Geometry: see drawing. Coordinates: mm, zero at the bounding-box minimum. Give positions to 0.01 mm unless a question says otherwise; leave off trailing zeros. Loops run counter-clockwise (first coordinate to the right, second up) from the corner with the lowest first, then second, coordinate; pieces in that order, holes last. Notation, with made-up numbers: (12.25, 66.25) -> (70.25, 66.25) arc R26 ccw to (70.25, 87.25) -> close; hole circle Ø5 at (67, 72). An arc over 180 degrees is marked (long way). One line per question, with ' | ' between items.
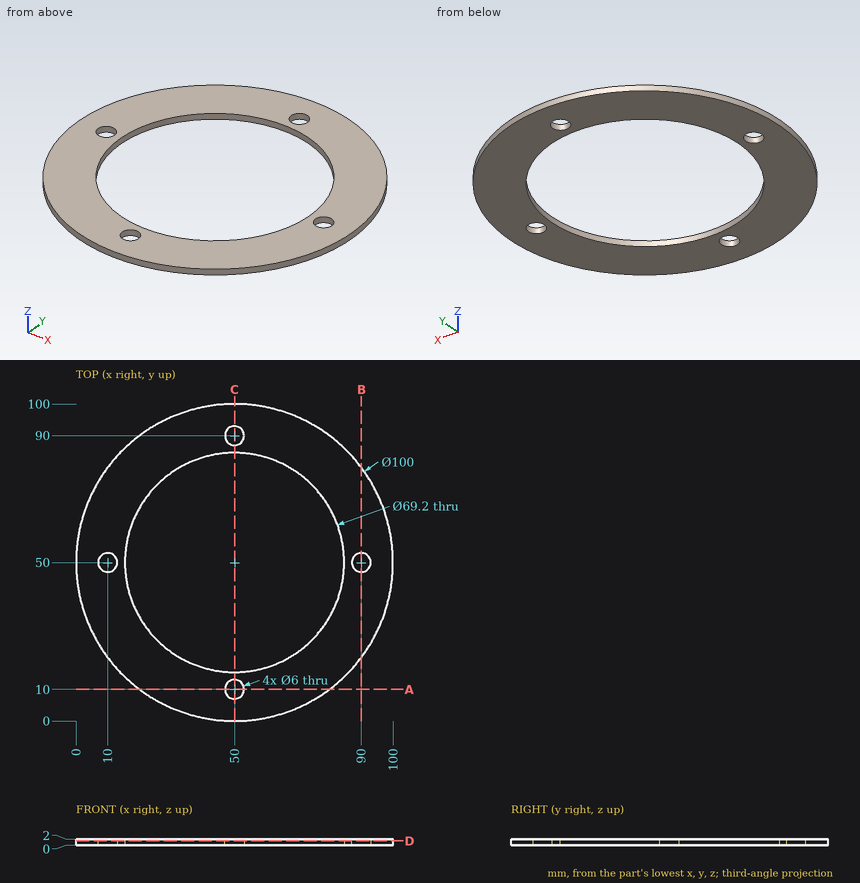
1. Ray query, line 1 along Y through (x, z) = (50, 1.65); line 2 along X through (y, z) = (49.5, 0.4); line 3 along Y through (x, z) = (33.5, 1.9). Return the intervals inside material, ascending. Write a range as from..to.
Determined:
line 1: y = 0..7, 13..15.4, 84.6..87, 93..100 | line 2: x = 0..7.04, 12.96..15.4, 84.6..87.04, 92.96..100 | line 3: y = 2.8..19.59, 80.41..97.2
2. Pin query (flat end, axial travel): P1, Ø4, axis at x = 38.5, y = 89, coming from the -Z side; P2, Ø3.5, axis at x = 10, y = 50, coming from the +Z side; P3, Ø1, axis at x = 17, z = 1, coming from the -Y side. Return the tip coordinate at first contact, or that it passes through.
Determined:
P1: stops at z = 0 | P2: passes through | P3: stops at y = 12
3. Section query A-A (y = 10). Output: boundary loops of the cut face in (x, z).
Determined:
outline: (20, 0) -> (47, 0) -> (47, 2) -> (20, 2) -> close; (53, 0) -> (80, 0) -> (80, 2) -> (53, 2) -> close
4. Section query C-C (x = 50). Output: boundary loops of the cut face in (y, z), then the cut area to 3 significant figures.
Determined:
outline: (0, 0) -> (7, 0) -> (7, 2) -> (0, 2) -> close; (13, 0) -> (15.4, 0) -> (15.4, 2) -> (13, 2) -> close; (84.6, 0) -> (87, 0) -> (87, 2) -> (84.6, 2) -> close; (93, 0) -> (100, 0) -> (100, 2) -> (93, 2) -> close | area: 37.6 mm2
5. Section query D-D (z = 1.4). Output: boundary loops of the cut face in (x, y), then the cut area to 3 significant figures.
Determined:
outline: circle Ø100 at (50, 50); hole circle Ø6 at (10, 50); hole circle Ø69.2 at (50, 50); hole circle Ø6 at (50, 10); hole circle Ø6 at (50, 90); hole circle Ø6 at (90, 50) | area: 3,980 mm2
